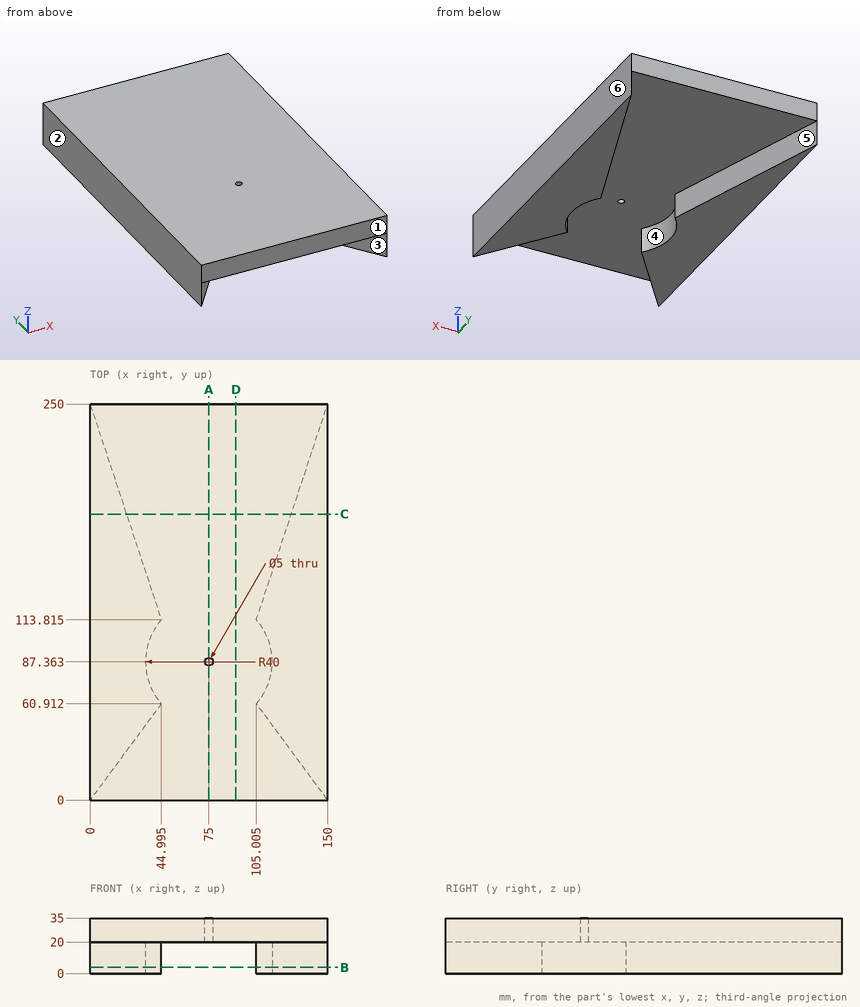
Input: dimensioned drawing with shaded views. Units: mm. Origin: part minimum x, y, z. A direction names the side the tool comes from. Coordinates: 2 decimals unless noted, no trailing zeros. Loops run counter-clockwise (first coordinate to the right, second up) from the corner with the lowest first, then second, coordinate; pieces in that order, holes last. Notation, with made-up numbers: (2.25, -2) -> (24.25, -2) arc R19 ccw to (24.25, 31) -> close; hole circle Ø6 at (-25, 48). An arc over 180 degrees is marked (long way). Use a Markdown table: item, result. Add a question column.
(1) Section query A-A, the plane x = 75. Return loops of the section in (y, z), plus the area to 4 significant figures.
(2) Access query for the marked faces 4, 5 and 6. Directions: +Z, -Z, +X, -X, +Y, -Y. A direction counts if a zero-diameter tool reaches every point of the face in a straight line with its end or side. Return the directions, or none.
(3) Pin query (flat end, axial travel): pin 1 Ø12 at (x, y) = (87, 56.5) entering from -Z; pin 2 Ø6 at (x, z) = (129.5, 9) entering from -Y. Return the tip coordinate at first contact, or that it passes through.
(4) Mould query, pull axis X, two halves, no side actions, for the marked faces 1, 2 and 3. Classes: pulls with the +X half, pulls with the -X half, needs draft (parallel to the pull), parting line crosses it, or undercut.
(5) Section query D-D, the plane x = 92. Return loops of the section in (y, z), plus the area to 3 significant figures.
(6) Section query B-B, the plane z = 4. Return loops of the section in (x, y) (1 decimal).
(7) Section query C-C, the plane y = 180.5. Return loops of the section in (x, z), plus the area to 3 significant figures.
(8) Line query: line 1 along Y through (x, z) = (75, 29); line 2 along Z through (x, y) = (88, 144); line 3 along X through (y, z) = (158, 13.5) (1 decimal). Output: solid intervals per line, ascending.
Answer:
| question | item | result |
|---|---|---|
| 1 | outline | (0, 20) -> (84.86, 20) -> (84.86, 35) -> (0, 35) -> close; (89.86, 20) -> (250, 20) -> (250, 35) -> (89.86, 35) -> close |
| 1 | area | 3,675 mm^2 |
| 2 | face 4 | -Z |
| 2 | face 5 | -Z, +Y |
| 2 | face 6 | +Z, -Z, +X, +Y, -Y |
| 3 | pin 1 | stops at z = 20 |
| 3 | pin 2 | stops at y = 23.69 |
| 4 | face 1 | needs draft |
| 4 | face 2 | pulls with the -X half |
| 4 | face 3 | undercut |
| 5 | outline | (0, 20) -> (250, 20) -> (250, 35) -> (0, 35) -> close |
| 5 | area | 3,750 mm^2 |
| 6 | outline | (0, 0) -> (45, 60.9) arc R40 cw to (45, 113.8) -> (0, 250) -> close; (105, 60.9) -> (150, 0) -> (150, 250) -> (105, 113.8) arc R40 cw to start |
| 7 | outline | (0, 0) -> (22.96, 0) -> (22.96, 20) -> (127.04, 20) -> (127.04, 0) -> (150, 0) -> (150, 35) -> (0, 35) -> close |
| 7 | area | 3,170 mm^2 |
| 8 | line 1 | y = 0 to 84.86, 89.86 to 250 |
| 8 | line 2 | z = 20 to 35 |
| 8 | line 3 | x = 0 to 30.4, 119.6 to 150 |
